```python
from build123d import *

# Parameters (mm, degrees)
F1_DEPTH = 60
F2_R     = 3
F3_R     = 3
F5_W     = 15
F5_H     = 8
F6_DEPTH = 25


with BuildPart() as f1:
    # F0 (on Right) → F1 (new body)
    with BuildSketch(Plane.YZ):
        Polygon((0, 0), (90, 0), (90, 10), (85, 10), (85, 5), (73.1801488287, 5), (45.2599553973, 81.7101009996), (40.5614915158, 80), (44.6500255673, 68.7668450149), (0, 5), align=None)
        Polygon((56.9401520578, 35), (67.8592590858, 5), (6.1038729438, 5), (27.583580996, 35.6762022401), (46.7376730664, 63.0310806514), align=None, mode=Mode.SUBTRACT)
    extrude(amount=F1_DEPTH)

    # F2
    f2_edges = [f1.edges().sort_by_distance(p)[0] for p in [
        (30, 6.103873, 5),
        (30, 67.859259, 5),
        (30, 46.737673, 63.031081),
        (30, 44.650026, 68.766845),
    ]]
    fillet(f2_edges, radius=F2_R)

    # F3
    f3_edges = [f1.edges().sort_by_distance(p)[0] for p in [
        (60, 42.910723, 80.85505),
        (0, 42.910723, 80.85505),
    ]]
    fillet(f3_edges, radius=F3_R)

    # F5 (on offset) → F6 (cut)
    with BuildSketch(Plane.XY.offset(5)):
        with Locations((30, 77.1801488287)):
            Rectangle(F5_W, F5_H)
    extrude(amount=-F6_DEPTH, mode=Mode.SUBTRACT)


solid = f1.part
```
Geometry: final body of the model. Coordinates: model frame, mm. A direction names the side the tool comes from. Coordinates: 2 decimals unless noted, no trailing zeros. Order: outer loops, then holes, each group sorted by start corner. A loop starts at its lowest first (then second) coordinate and runs counter-clockwise, first axis right, second up. Notation, with made-up numbers: (-36.75, 34) -> (19.25, 34) arc R25 ccw to (19.25, 70) -> close; hole circle Ø6 at (46, 21.5). An arc over 180 degrees is marked (long way). Answer in a Markdown table with one row per item.
Item 1: Section A-A on z = 24. Output: boundary loops of the cut face in (x, y), plus the area to 3 significant figures.
Return value:
| item | result |
|---|---|
| outline | (0, 13.3) -> (60, 13.3) -> (60, 19.41) -> (0, 19.41) -> close; (0, 60.94) -> (60, 60.94) -> (60, 66.26) -> (0, 66.26) -> close |
| area | 685 mm² |
Item 2: Ray query, L1, parallel to Y at x = 57.5, z = 24.5; L2, parallel to Y at x = 25, z = 9; L3, parallel to Z at x = 9, y = 76. Return the intervals inside material, ascending.
Return value:
| item | result |
|---|---|
| L1 | y = 13.65 to 19.76, 60.76 to 66.08 |
| L2 | y = 2.8 to 9.04, 66.4 to 71.72, 85 to 90 |
| L3 | z = 0 to 5 |
Item 3: Access query for faces 1 (the flat face through (30, 82, 5)), 2 (the flat face through (30, 73.18, 3)), 3 (the cylindrical face through (30.42, 9.23, 6.57)), 4 (the flat face through (30, 88, 10)). Directions: +Z, -Z, +X, -X, +Y, -Y. A direction counts if a zero-diameter tool reaches every point of the face in a straight line with its end or side. Return the directions, or none.
Return value:
| item | result |
|---|---|
| face 1 | +Z, +X, -X |
| face 2 | +Z, -Z |
| face 3 | +X, -X |
| face 4 | +Z, +X, -X, +Y |
Item 4: Section C-C on x = 54. Output: boundary loops of the cut face in (y, z).
Return value:
| item | result |
|---|---|
| outline | (0, 0) -> (90, 0) -> (90, 10) -> (85, 10) -> (85, 5) -> (73.18, 5) -> (45.26, 81.71) -> (40.56, 80) -> (44.12, 70.23) arc R3 cw to (43.75, 67.49) -> (0, 5) -> close; hole (9.41, 9.72) arc R3 ccw to (11.87, 5) -> (63.57, 5) arc R3 ccw to (66.39, 9.03) -> (48.71, 57.62) arc R3 ccw to (43.43, 58.31) -> close |
Item 5: Draft query along Z for faces 5 (the flat face through (29.58, 42.314, 75.186)), 6 (the cylindrical face through (59.098, 43.17, 80.039)), 7 (the flat face through (37.5, 77, 3)). Return one class per face: released by +Z, released by -Z, zero draft, split by the parting line, or undercut.
Return value:
| item | result |
|---|---|
| face 5 | undercut |
| face 6 | released by +Z |
| face 7 | zero draft |
Item 6: Contact query for flat-ended pins moving along their axis: P1, Ø4, axis at y = 38.5, z = 66.5, coming from the -X side; P2, Ø12, axis at x = 17.5, z = 60.5, coming from the +Y side; P3, Ø1.5, axis at x = 36.5, y = 88, coming from the +Z side; P4, Ø4, axis at x = 40.5, z = 8, coming from the -Y side. Output: stop coordinate, or through.
Return value:
| item | result |
|---|---|
| P1 | passes through |
| P2 | stops at y = 55.16 |
| P3 | stops at z = 10 |
| P4 | stops at y = 0.7 |
Item 7: Section B-B on y = 50. Output: boundary loops of the cut face in (x, z), plus the area to 3 significant figures.
Return value:
| item | result |
|---|---|
| outline | (0, 0) -> (60, 0) -> (60, 5) -> (0, 5) -> close; (0, 54.07) -> (60, 54.07) -> (60, 68.69) -> (0, 68.69) -> close |
| area | 1,180 mm² |
Item 8: Section D-D on z = 61. Output: boundary loops of the cut face in (x, y).
Return value:
| item | result |
|---|---|
| outline | (0, 39.21) -> (60, 39.21) -> (60, 52.8) -> (0, 52.8) -> close |
